Geometry check sheet. Reference: the model listing, model coordinates, mm. A direction names the side the tool comes from. Coordinates: 2 decimals unless noted, no trailing zeros. Loops run counter-clockwise (first coordinate to the right, second up) from the corner with the lowest first, then second, coordinate; pieces in that order, holes last.
from build123d import *

# Parameters (mm, degrees)
SKETCH1_R           = 3
BOSS_EXTRUDE1_DEPTH = 3
SKETCH2_R           = 7
SKETCH2_R_2         = 3
BOSS_EXTRUDE2_DEPTH = 3
CHAMFER1_SIZE       = 0.5


with BuildPart() as part:
    # Sketch1 → Boss-Extrude1 (new body)
    with BuildSketch(Plane(origin=(0, 0, 0), x_dir=(1, 0, 0), z_dir=(0, 1, 0))):
        with BuildLine():
            ThreePointArc((9.090097423, 5.554563517), (5.554563517, 5.554563517), (5.554563517, 9.090097423))
            Line((5.554563517, 9.090097423), (15.821292146, 19.356826052))
            ThreePointArc((15.821292146, 19.356826052), (14.892716162, 20.080015073), (13.931131824, 20.758698564))
            ThreePointArc((13.931131824, 20.758698564), (0, 15.17766953), (-13.931131824, 20.758698564))
            ThreePointArc((-13.931131824, 20.758698564), (-14.892716162, 20.080015073), (-15.821292146, 19.356826052))
            Line((-15.821292146, 19.356826052), (-5.554563517, 9.090097423))
            ThreePointArc((-5.554563517, 9.090097423), (-5.554563517, 5.554563517), (-9.090097423, 5.554563517))
            Line((-9.090097423, 5.554563517), (-19.356826052, 15.821292146))
            ThreePointArc((-19.356826052, 15.821292146), (-20.080015073, 14.892716162), (-20.758698564, 13.931131824))
            ThreePointArc((-20.758698564, 13.931131824), (-15.17766953, 0), (-20.758698564, -13.931131824))
            ThreePointArc((-20.758698564, -13.931131824), (-20.080015073, -14.892716162), (-19.356826052, -15.821292146))
            Line((-19.356826052, -15.821292146), (-9.090097423, -5.554563517))
            ThreePointArc((-9.090097423, -5.554563517), (-5.554563517, -5.554563517), (-5.554563517, -9.090097423))
            Line((-5.554563517, -9.090097423), (-15.821292146, -19.356826052))
            ThreePointArc((-15.821292146, -19.356826052), (-14.892716162, -20.080015073), (-13.931131824, -20.758698564))
            ThreePointArc((-13.931131824, -20.758698564), (0, -15.17766953), (13.931131824, -20.758698564))
            ThreePointArc((13.931131824, -20.758698564), (14.892716162, -20.080015073), (15.821292146, -19.356826052))
            Line((15.821292146, -19.356826052), (5.554563517, -9.090097423))
            ThreePointArc((5.554563517, -9.090097423), (5.554563517, -5.554563517), (9.090097423, -5.554563517))
            Line((9.090097423, -5.554563517), (19.356826052, -15.821292146))
            ThreePointArc((19.356826052, -15.821292146), (20.080015073, -14.892716162), (20.758698564, -13.931131824))
            ThreePointArc((20.758698564, -13.931131824), (15.17766953, 0), (20.758698564, 13.931131824))
            ThreePointArc((20.758698564, 13.931131824), (20.080015073, 14.892716162), (19.356826052, 15.821292146))
            Line((19.356826052, 15.821292146), (9.090097423, 5.554563517))
        make_face()
        with Locations(Location((0, 0, 0), (0, 0, 270))):
            Circle(SKETCH1_R, mode=Mode.SUBTRACT)
    extrude(amount=BOSS_EXTRUDE1_DEPTH)

    # Sketch2 → Boss-Extrude2 (add)
    with BuildSketch(Plane(origin=(0, 3, 0), x_dir=(1, 0, 0), z_dir=(0, 1, 0))):
        with Locations(Location((0, 0, 0), (0, 0, 270))):
            Circle(SKETCH2_R)
        with Locations(Location((0, 0, 0), (0, 0, 270))):
            Circle(SKETCH2_R_2, mode=Mode.SUBTRACT)
    extrude(amount=BOSS_EXTRUDE2_DEPTH)

    # Chamfer1
    chamfer1_edges = [part.edges().sort_by_distance(p)[0] for p in [
        (0, 6, -7),
        (10.687927832, 3, 14.223461738),
        (5.554563517, 3, 5.554563517),
        (14.223461738, 3, 10.687927832),
        (20.080015073, 3, 14.892716162),
        (15.17766953, 3, 0),
        (20.080015073, 3, -14.892716162),
        (14.223461738, 3, -10.687927832),
        (5.554563517, 3, -5.554563517),
        (10.687927832, 3, -14.223461738),
        (0, 3, 15.17766953),
        (-14.892716162, 3, 20.080015073),
        (-10.687927832, 3, 14.223461738),
        (-5.554563517, 3, 5.554563517),
        (-14.223461738, 3, 10.687927832),
        (-20.080015073, 3, 14.892716162),
        (-15.17766953, 3, 0),
        (-20.080015073, 3, -14.892716162),
        (0, 3, -15.17766953),
        (-14.892716162, 3, -20.080015073),
        (-10.687927832, 3, -14.223461738),
        (-5.554563517, 3, -5.554563517),
        (-14.223461738, 3, -10.687927832),
        (0, 6, -3),
        (0, 0, -3),
        (20.080015073, 0, 14.892716162),
        (14.223461738, 0, 10.687927832),
        (5.554563517, 0, 5.554563517),
        (10.687927832, 0, 14.223461738),
        (14.892716162, 0, 20.080015073),
        (0, 0, 15.17766953),
        (-14.892716162, 0, 20.080015073),
        (-10.687927832, 0, 14.223461738),
        (-5.554563517, 0, 5.554563517),
        (-14.223461738, 0, 10.687927832),
        (-20.080015073, 0, 14.892716162),
        (-15.17766953, 0, 0),
        (-20.080015073, 0, -14.892716162),
        (-14.223461738, 0, -10.687927832),
        (-5.554563517, 0, -5.554563517),
        (-10.687927832, 0, -14.223461738),
        (-14.892716162, 0, -20.080015073),
        (0, 0, -15.17766953),
        (14.892716162, 0, -20.080015073),
        (10.687927832, 0, -14.223461738),
        (5.554563517, 0, -5.554563517),
        (14.223461738, 0, -10.687927832),
        (20.080015073, 0, -14.892716162),
        (15.17766953, 0, 0),
    ]]
    chamfer(chamfer1_edges, length=CHAMFER1_SIZE)


solid = part.part
(1) Gauge pin test, flat ends, axial feed: pin 1 Ø10 at (x, z) = (-1.5, 14.5) entering from +Y; pin 2 Ø1 at (x, y) = (4.5, 2.5) entering from -Z. Record the tip position at first contact, or that the pin passes through.
Findings:
pin 1: stops at y = 3
pin 2: stops at z = -15.81
(2) Access from +Z, -Z, +X, -X, +Y, -Y to the whole of each face (thin tool, end or side, straight path). Record for faces 1 (the flat face through (10.616, 1.486, -14.152)), 2 (the flat face through (-14.47, 2.75, 10.58)), 3 (the flat face through (14.47, 0.253, -10.585)).
Findings:
face 1: +Y, -Y
face 2: +Y
face 3: -Y
(3) Sectioned sample at C-C on x = 0. Record the cut outline in (y, z).
Findings:
outline: (0, -14.68) - (0.5, -15.18) - (2.5, -15.18) - (3, -14.68) - (3, -7) - (5.5, -7) - (6, -6.5) - (6, -3.5) - (5.5, -3) - (0.5, -3) - (0, -3.5) - close; (0, 3.5) - (0.5, 3) - (5.5, 3) - (6, 3.5) - (6, 6.5) - (5.5, 7) - (3, 7) - (3, 14.68) - (2.5, 15.18) - (0.5, 15.18) - (0, 14.68) - close
(4) Draft check along X on faces 4 (the flat face through (-9, 3, 0)), 5 (the conical face through (-14.73, 2.75, -19.89)), 6 (the flat face through (10.76, 1.486, 14.295)), 7 (the conical face through (-5.41, 2.64, -5.5)). Enter one of: +X half, -X half, draft (parallel to the pull), parting line (faces both ways), or undercut.
Findings:
face 4: draft
face 5: -X half
face 6: undercut
face 7: undercut
(5) Sectioned sample at A-A on z = 0. Record the cut outline in (x, y).
Findings:
outline: (-15.18, 0.5) - (-14.68, 0) - (-3.5, 0) - (-3, 0.5) - (-3, 5.5) - (-3.5, 6) - (-6.5, 6) - (-7, 5.5) - (-7, 3) - (-14.68, 3) - (-15.18, 2.5) - close; (3, 0.5) - (3.5, 0) - (14.68, 0) - (15.18, 0.5) - (15.18, 2.5) - (14.68, 3) - (7, 3) - (7, 5.5) - (6.5, 6) - (3.5, 6) - (3, 5.5) - close
(6) Scan lines: L1, parallel to X at y = 4.2, z = 0; L2, parallel to Y at x = 10.5, z = -16; L3, parallel to Z at x = 14, y = 0.75. Record each from-to range of solid material in increasing order.
Findings:
L1: x = -7 to -3, 3 to 7
L2: y = 0 to 3
L3: z = -20.71 to -17.54, -10.46 to 10.46, 17.54 to 20.71
(7) Sectioned sample at D-D on x = 7.5. State how many separate pieces and enclosed holes the cut face has, and give its area (3 significant figures).
Findings:
separate pieces: 3
enclosed holes: 0
area: 60.8 mm2
(8) Sectioned sample at B-B on y = 1.75. Record the cut outline in (x, z).
Findings:
outline: (-20.76, -13.93) arc R25 ccw to (-19.36, -15.82) - (-9.09, -5.55) arc R2.5 cw to (-5.55, -9.09) - (-15.82, -19.36) arc R25 ccw to (-13.93, -20.76) arc R20.18 cw to (13.93, -20.76) arc R25 ccw to (15.82, -19.36) - (5.55, -9.09) arc R2.5 cw to (9.09, -5.55) - (19.36, -15.82) arc R25 ccw to (20.76, -13.93) arc R20.18 cw to (20.76, 13.93) arc R25 ccw to (19.36, 15.82) - (9.09, 5.55) arc R2.5 cw to (5.55, 9.09) - (15.82, 19.36) arc R25 ccw to (13.93, 20.76) arc R20.18 cw to (-13.93, 20.76) arc R25 ccw to (-15.82, 19.36) - (-5.55, 9.09) arc R2.5 cw to (-9.09, 5.55) - (-19.36, 15.82) arc R25 ccw to (-20.76, 13.93) arc R20.18 cw to start; hole circle Ø6 at (0, 0)
